Geometry: see drawing. Coordinates: mm, zero at the bounding-box minimum. Give positions to 0.01 mm unless a question says otherwise; leave off trailing zeros. Order: outer loops, then holes, each group sorted by start corner. A loop starts at its lowest first (then second) coordinate and runs counter-clockwise, first axis right, second up. Notation, with made-up numbers: (7.5, -32) - (25.5, -32) arc R23 cw to (25.5, -14) - close; hole circle Ø4 at (55.25, 17). An arc over 180 degrees is marked (long way). One line per item, written item: value.
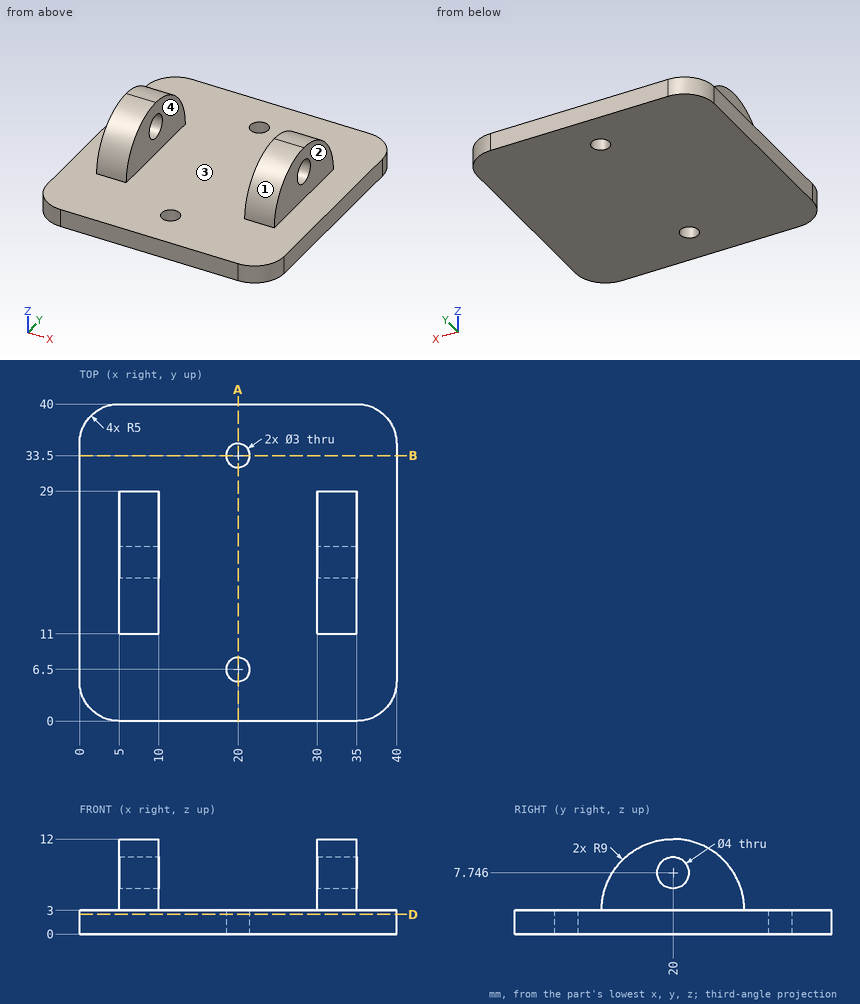
1) Section B-B, the plane y = 33.5. Return loops of the section in (x, z).
Answers below:
outline: (0, 0) - (18.5, 0) - (18.5, 3) - (0, 3) - close; (21.5, 0) - (40, 0) - (40, 3) - (21.5, 3) - close
2) First-contact query: pin 1 (3 mm diameter, centred on y = 20, z = 7.75, fed in from -X); pin 2 (4.5 mm diameter, centred on y = 20, z = 7.75, fed in from -X); pin 3 (2.5 mm diameter, centred on y = 16.5, z = 9.5, fed in from +X); pin 4 (3 mm diameter, centred on x = 18.5, y = 25, fed in from +Z). Flat tips, straight axial feed; report the tip coordinate or a pass-through.
Answers below:
pin 1: through
pin 2: x = 5
pin 3: x = 35
pin 4: z = 3
3) Material intervals for line 1 along X through (y, z) = (16.5, 7); line 2 along Z through (x, y) = (16.5, 26.5); line 3 along Y through (x, z) = (5.5, 10.75) (1 decimal), sorted ascending.
Answers below:
line 1: 5 to 10, 30 to 35
line 2: 0 to 3
line 3: 15.4 to 24.6
4) Mould query, pull axis X, two halves, no side actions, for the marked faces 1, 2, 3 and 4. Classes: released by +X, released by -X, zero draft, split by the parting line, or undercut.
Answers below:
face 1: zero draft
face 2: released by +X
face 3: undercut
face 4: undercut
5) Section A-A, the plane x = 20. Return loops of the section in (y, z), then the cut area to 3 significant figures.
Answers below:
outline: (0, 0) - (5, 0) - (5, 3) - (0, 3) - close; (8, 0) - (32, 0) - (32, 3) - (8, 3) - close; (35, 0) - (40, 0) - (40, 3) - (35, 3) - close
area: 102 mm^2
6) Section D-D, the plane z = 2.5. Return loops of the section in (x, y), then the cut area to 3 significant figures.
Answers below:
outline: (0, 5) arc R5 ccw to (5, 0) - (35, 0) arc R5 ccw to (40, 5) - (40, 35) arc R5 ccw to (35, 40) - (5, 40) arc R5 ccw to (0, 35) - close; hole circle Ø3 at (20, 6.5); hole circle Ø3 at (20, 33.5)
area: 1,560 mm^2
